The listing builds one solid part. Answer for the finished solid, in the listing's coordinates (mm). Face numbers are marked on the shaded views. A direction names the side the tool comes from. Round coordinates to 2 decimals unless told otherwise and drop trailing zeros. Loops run counter-clockwise (first coordinate to the right, second up) from the corner with the lowest first, then second, coordinate; pieces in that order, holes last. Notation, with made-up numbers: (27, -28) - (34, -28) arc R23 ccw to (34, -15) - close; hole circle Ø2 at (-27.5, -34). An arc over 180 degrees is marked (long way). Write item = value, one per line. Start each with the question number.
1) Section A-A, the plane x = 0 is taken. Determine the outline of the cut face in (y, z).
2) Given pin 1 Ø5 at (x, z) = (-8, 4.5) entering from -Y; pin 2 Ø2 at (y, z) = (8.5, 7.5) entering from -X; pin 3 Ø6 at (y, z) = (3, 4.5) entering from -X, each flat-ended and moving along its own axis, determine where each tip first touches the part or whether it passes through.
3) A tool of negligible diameter and unlimited length cuts with its end or side. For the marked faces 4 and 5, from which of +Z, -Z, +X, -X, +Y, -Y can it reach the whole face along a straight path? Write none if from no direction.
4) Straight lines are drawn through the part: line 1 along Y through (x, z) = (0, 7); line 2 along X through (y, z) = (-7.25, 5.75); line 3 along Y through (x, z) = (-14, 3). For each, find the intervals that lie inside material, in ascending order.
5) Section C-C, the plane z = 1 is taken. Determine the outline of the cut face in (x, y).
6) Section B-B, the plane y = 8.5 is taken. Determine the outline of the cut face in (x, z).
7) For a pull along X with two mould halves and no side action, classify the marked faces 1, 2 and 3 as released by +X, released by -X, zero draft, split by the parting line, or undercut.
8) Section D-D, the plane y = -2 is taken. Determine the outline of the cut face in (x, z).
from build123d import *

# Parameters (mm, degrees)
AUFSATZ_LINEAR_AUSTRAGEN3_DEPTH      = 20
SKIZZE10_OUTSIDE_W                   = 46.486
SKIZZE10_OUTSIDE_H                   = 31.486
SCHNITT_LINEAR_AUSTRAGEN9_DEPTH      = 13.5
SCHNITT_LINEAR_AUSTRAGEN9_DEPTH_BACK = 13.5
SKIZZE7_R                            = 1.23
SCHNITT_LINEAR_AUSTRAGEN8_DEPTH      = 12


with BuildPart() as part:
    # Skizze3 → Aufsatz-Linear austragen3 (new body)
    with BuildSketch(Plane.XY):
        with BuildLine():
            Line((-17.5, 4), (-2.314936357, 11.931824643))
            ThreePointArc((-2.314936357, 11.931824643), (0, 12.5), (2.314936357, 11.931824643))
            Line((2.314936357, 11.931824643), (17.5, 4))
            Line((17.5, 4), (17.5, -4))
            Line((17.5, -4), (2.314936357, -11.931824643))
            ThreePointArc((2.314936357, -11.931824643), (0, -12.5), (-2.314936357, -11.931824643))
            Line((-2.314936357, -11.931824643), (-17.5, -4))
            Line((-17.5, -4), (-17.5, 4))
        make_face()
        with BuildLine():
            Line((-2.25, -7.5), (-2.25, 7.5))
            ThreePointArc((-2.25, 7.5), (0, 9.75), (2.25, 7.5))
            Line((2.25, 7.5), (2.25, -7.5))
            ThreePointArc((2.25, -7.5), (0, -9.75), (-2.25, -7.5))
        make_face(mode=Mode.SUBTRACT)
    extrude(amount=AUFSATZ_LINEAR_AUSTRAGEN3_DEPTH)

    # Skizze10 outside → Schnitt-Linear austragen9 (cut, two sides)
    with BuildSketch(Plane(origin=(0, 0, 0), x_dir=(1, 0, 0), z_dir=(0, 1, 0))) as schnitt_linear_austragen9_sk:
        with Locations((0, -10)):
            Rectangle(SKIZZE10_OUTSIDE_W, SKIZZE10_OUTSIDE_H)
        with BuildLine():
            Line((-16.455790462, 0), (-17.5, -7.931558891))
            Line((-17.5, -7.931558891), (-2.610523844, -9.891795615))
            ThreePointArc((-2.610523844, -9.891795615), (0, -10.062898387), (2.610523844, -9.891795615))
            Line((2.610523844, -9.891795615), (17.5, -7.931558891))
            Line((17.5, -7.931558891), (16.455790462, 0))
            Line((16.455790462, 0), (-16.455790462, 0))
        make_face(mode=Mode.SUBTRACT)
    extrude(amount=SCHNITT_LINEAR_AUSTRAGEN9_DEPTH, mode=Mode.SUBTRACT)
    extrude(schnitt_linear_austragen9_sk.sketch, amount=-SCHNITT_LINEAR_AUSTRAGEN9_DEPTH_BACK, mode=Mode.SUBTRACT)

    # Skizze7 → Schnitt-Linear austragen8 (cut)
    with BuildSketch(Plane(origin=(-17.19638108, 0, 5.625344227), x_dir=(-0.130526192, 0, 0.991444861), z_dir=(-0.991444861, 0, -0.130526192))):
        with Locations((-2.173885101, 0)):
            Circle(SKIZZE7_R)
    schnitt_linear_austragen8 = extrude(amount=-SCHNITT_LINEAR_AUSTRAGEN8_DEPTH, mode=Mode.SUBTRACT)

    # Spiegeln4: Schnitt-Linear austragen8 across plane
    add(schnitt_linear_austragen8.mirror(Plane(origin=(0, 0, 0), x_dir=(0, 0, 1), z_dir=(1, 0, 0))), mode=Mode.SUBTRACT)


solid = part.part
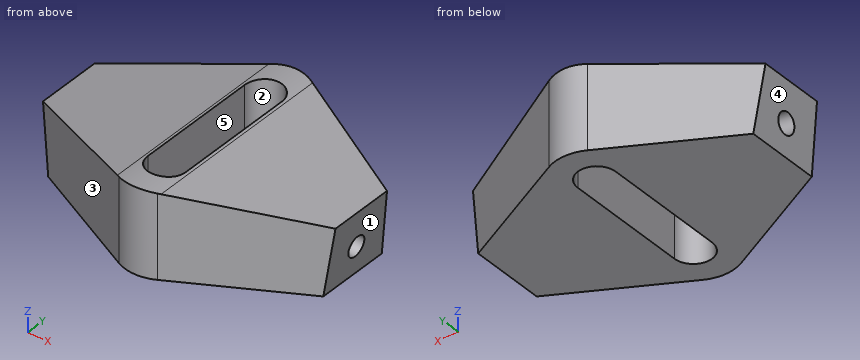
Geometry check:
q1.outline = (-12.5, 0) - (-9.75, 0) - (-9.75, 10.06) - (-12.5, 10.06) - close; (9.75, 0) - (12.5, 0) - (12.5, 10.06) - (9.75, 10.06) - close
q2.pin_1 = -10.27
q2.pin_2 = -10.8
q2.pin_3 = -17.44
q3.face_4 = -Z, -X, +Y, -Y
q3.face_5 = +Z, -Z
q4.line_1 = -12.5 to -9.75, 9.75 to 12.5
q4.line_2 = -11.28 to -2.25, 2.25 to 11.28
q4.line_3 = -5.83 to -0.89, 0.89 to 5.83
q5.outline = (-16.59, -4.48) - (-2.31, -11.93) arc R5 ccw to (2.31, -11.93) - (16.59, -4.48) - (16.59, 4.48) - (2.31, 11.93) arc R5 ccw to (-2.31, 11.93) - (-16.59, 4.48) - close; hole (-2.25, -7.5) arc R2.25 ccw to (2.25, -7.5) - (2.25, 7.5) arc R2.25 ccw to (-2.25, 7.5) - close
q6.outline = (-8.88, 0) - (-2.02, 0) - (-2.02, 9.96) arc R20 ccw to (-2.61, 9.89) - (-8.88, 9.07) - close; (2.02, 0) - (8.88, 0) - (8.88, 9.07) - (2.61, 9.89) arc R20 ccw to (2.02, 9.96) - close
q7.face_1 = released by +X
q7.face_2 = undercut
q7.face_3 = released by -X
q8.outline = (-17.5, 7.93) - (-16.46, 0) - (-2.25, 0) - (-2.25, 9.94) arc R20 ccw to (-2.61, 9.89) - close; (2.25, 0) - (16.46, 0) - (17.5, 7.93) - (2.61, 9.89) arc R20 ccw to (2.25, 9.94) - close
